```python
from build123d import *

# Parameters (mm, degrees)
BOSS_EXTRUDE1_DEPTH = 37
CUT_EXTRUDE1_REACH  = 186.762
SKETCH2_R           = 11.5
CUT_EXTRUDE2_REACH  = 186.762
SKETCH3_R           = 1.25
SKETCH5_W           = 38
SKETCH5_H           = 23
CUT_EXTRUDE3_DEPTH  = 3
SKETCH6_W           = 3
SKETCH6_H           = 23
BOSS_EXTRUDE2_DEPTH = 7.5
CUT_EXTRUDE4_REACH  = 184.696
SKETCH7_R           = 1.25
SKETCH8_R           = 2.05
CUT_EXTRUDE5_DEPTH  = 2
CUT_EXTRUDE6_REACH  = 181.313
SKETCH9_R           = 2.25
SKETCH10_R          = 3.6
CUT_EXTRUDE7_DEPTH  = 4
CHAMFER1_SIZE       = 30
FILLET4_R           = 20


with BuildPart() as part:
    # Sketch1 → Boss-Extrude1 (new body)
    with BuildSketch(Plane(origin=(0, 0, 0), x_dir=(1, 0, 0), z_dir=(0, 1, 0))):
        Polygon((0, 0), (0, 128), (128, 128), (128, 120), (8, 120), (8, 0), align=None)
    extrude(amount=BOSS_EXTRUDE1_DEPTH)

    # Sketch2 → Cut-Extrude1 (cut, up to next)
    with BuildSketch(Plane(origin=(0, 0, -128), x_dir=(-1, 0, 0), z_dir=(0, 0, -1)), mode=Mode.PRIVATE) as cut_extrude1_sk1:
        with Locations((-112, 18.5)):
            Circle(SKETCH2_R)
    cut_extrude1_tool1 = extrude(cut_extrude1_sk1.sketch, amount=-CUT_EXTRUDE1_REACH, mode=Mode.PRIVATE) & part.part
    add(cut_extrude1_tool1.solids().sort_by_distance((112, 18.5, -128))[0], mode=Mode.SUBTRACT)

    # Sketch3 → Cut-Extrude2 (cut, up to next)
    with BuildSketch(Plane(origin=(0, 0, -128), x_dir=(-1, 0, 0), z_dir=(0, 0, -1)), mode=Mode.PRIVATE) as cut_extrude2_sk1:
        with Locations((-75.86, 10.31)):
            Circle(SKETCH3_R)
    cut_extrude2_tool1 = extrude(cut_extrude2_sk1.sketch, amount=-CUT_EXTRUDE2_REACH, mode=Mode.PRIVATE) & part.part
    # Sketch3 → Cut-Extrude2 (cut, up to next)
    with BuildSketch(Plane(origin=(0, 0, -128), x_dir=(-1, 0, 0), z_dir=(0, 0, -1)), mode=Mode.PRIVATE) as cut_extrude2_sk2:
        with Locations((-105.36, 32.19)):
            Circle(SKETCH3_R)
    cut_extrude2_tool2 = extrude(cut_extrude2_sk2.sketch, amount=-CUT_EXTRUDE2_REACH, mode=Mode.PRIVATE) & part.part
    # Sketch3 → Cut-Extrude2 (cut, up to next)
    with BuildSketch(Plane(origin=(0, 0, -128), x_dir=(-1, 0, 0), z_dir=(0, 0, -1)), mode=Mode.PRIVATE) as cut_extrude2_sk3:
        with Locations((-97.36, 32.19)):
            Circle(SKETCH3_R)
    cut_extrude2_tool3 = extrude(cut_extrude2_sk3.sketch, amount=-CUT_EXTRUDE2_REACH, mode=Mode.PRIVATE) & part.part
    # Sketch3 → Cut-Extrude2 (cut, up to next)
    with BuildSketch(Plane(origin=(0, 0, -128), x_dir=(-1, 0, 0), z_dir=(0, 0, -1)), mode=Mode.PRIVATE) as cut_extrude2_sk4:
        with Locations((-89.36, 32.19)):
            Circle(SKETCH3_R)
    cut_extrude2_tool4 = extrude(cut_extrude2_sk4.sketch, amount=-CUT_EXTRUDE2_REACH, mode=Mode.PRIVATE) & part.part
    # Sketch3 → Cut-Extrude2 (cut, up to next)
    with BuildSketch(Plane(origin=(0, 0, -128), x_dir=(-1, 0, 0), z_dir=(0, 0, -1)), mode=Mode.PRIVATE) as cut_extrude2_sk5:
        with Locations((-81.36, 32.19)):
            Circle(SKETCH3_R)
    cut_extrude2_tool5 = extrude(cut_extrude2_sk5.sketch, amount=-CUT_EXTRUDE2_REACH, mode=Mode.PRIVATE) & part.part
    # Sketch3 → Cut-Extrude2 (cut, up to next)
    with BuildSketch(Plane(origin=(0, 0, -128), x_dir=(-1, 0, 0), z_dir=(0, 0, -1)), mode=Mode.PRIVATE) as cut_extrude2_sk6:
        with Locations((-81.36, 4.81)):
            Circle(SKETCH3_R)
    cut_extrude2_tool6 = extrude(cut_extrude2_sk6.sketch, amount=-CUT_EXTRUDE2_REACH, mode=Mode.PRIVATE) & part.part
    # Sketch3 → Cut-Extrude2 (cut, up to next)
    with BuildSketch(Plane(origin=(0, 0, -128), x_dir=(-1, 0, 0), z_dir=(0, 0, -1)), mode=Mode.PRIVATE) as cut_extrude2_sk7:
        with Locations((-89.36, 4.81)):
            Circle(SKETCH3_R)
    cut_extrude2_tool7 = extrude(cut_extrude2_sk7.sketch, amount=-CUT_EXTRUDE2_REACH, mode=Mode.PRIVATE) & part.part
    # Sketch3 → Cut-Extrude2 (cut, up to next)
    with BuildSketch(Plane(origin=(0, 0, -128), x_dir=(-1, 0, 0), z_dir=(0, 0, -1)), mode=Mode.PRIVATE) as cut_extrude2_sk8:
        with Locations((-97.36, 4.81)):
            Circle(SKETCH3_R)
    cut_extrude2_tool8 = extrude(cut_extrude2_sk8.sketch, amount=-CUT_EXTRUDE2_REACH, mode=Mode.PRIVATE) & part.part
    # Sketch3 → Cut-Extrude2 (cut, up to next)
    with BuildSketch(Plane(origin=(0, 0, -128), x_dir=(-1, 0, 0), z_dir=(0, 0, -1)), mode=Mode.PRIVATE) as cut_extrude2_sk9:
        with Locations((-105.36, 4.81)):
            Circle(SKETCH3_R)
    cut_extrude2_tool9 = extrude(cut_extrude2_sk9.sketch, amount=-CUT_EXTRUDE2_REACH, mode=Mode.PRIVATE) & part.part
    # Sketch3 → Cut-Extrude2 (cut, up to next)
    with BuildSketch(Plane(origin=(0, 0, -128), x_dir=(-1, 0, 0), z_dir=(0, 0, -1)), mode=Mode.PRIVATE) as cut_extrude2_sk10:
        with Locations((-75.86, 26.69)):
            Circle(SKETCH3_R)
    cut_extrude2_tool10 = extrude(cut_extrude2_sk10.sketch, amount=-CUT_EXTRUDE2_REACH, mode=Mode.PRIVATE) & part.part
    add(cut_extrude2_tool1.solids().sort_by_distance((75.86, 10.31, -128))[0], mode=Mode.SUBTRACT)
    add(cut_extrude2_tool2.solids().sort_by_distance((105.36, 32.19, -128))[0], mode=Mode.SUBTRACT)
    add(cut_extrude2_tool3.solids().sort_by_distance((97.36, 32.19, -128))[0], mode=Mode.SUBTRACT)
    add(cut_extrude2_tool4.solids().sort_by_distance((89.36, 32.19, -128))[0], mode=Mode.SUBTRACT)
    add(cut_extrude2_tool5.solids().sort_by_distance((81.36, 32.19, -128))[0], mode=Mode.SUBTRACT)
    add(cut_extrude2_tool6.solids().sort_by_distance((81.36, 4.81, -128))[0], mode=Mode.SUBTRACT)
    add(cut_extrude2_tool7.solids().sort_by_distance((89.36, 4.81, -128))[0], mode=Mode.SUBTRACT)
    add(cut_extrude2_tool8.solids().sort_by_distance((97.36, 4.81, -128))[0], mode=Mode.SUBTRACT)
    add(cut_extrude2_tool9.solids().sort_by_distance((105.36, 4.81, -128))[0], mode=Mode.SUBTRACT)
    add(cut_extrude2_tool10.solids().sort_by_distance((75.86, 26.69, -128))[0], mode=Mode.SUBTRACT)

    # Sketch5 → Cut-Extrude3 (cut)
    with BuildSketch(Plane(origin=(0, 0, -128), x_dir=(-1, 0, 0), z_dir=(0, 0, -1))):
        with Locations((-90, 18.5)):
            Rectangle(SKETCH5_W, SKETCH5_H)
    extrude(amount=-CUT_EXTRUDE3_DEPTH, mode=Mode.SUBTRACT)

    # Sketch6 → Boss-Extrude2 (add)
    with BuildSketch(Plane(origin=(71, 0, 0), x_dir=(0, 0, -1), z_dir=(1, 0, 0))):
        with Locations((126.5, 18.5)):
            Rectangle(SKETCH6_W, SKETCH6_H)
    extrude(amount=BOSS_EXTRUDE2_DEPTH)

    # Sketch7 → Cut-Extrude4 (cut, up to next)
    with BuildSketch(Plane.XY.offset(-125), mode=Mode.PRIVATE) as cut_extrude4_sk1:
        with Locations(Location((75.86, 10.31, 0), (0, 0, 180))):
            Circle(SKETCH7_R)
    cut_extrude4_tool1 = extrude(cut_extrude4_sk1.sketch, amount=-CUT_EXTRUDE4_REACH, mode=Mode.PRIVATE) & part.part
    # Sketch7 → Cut-Extrude4 (cut, up to next)
    with BuildSketch(Plane.XY.offset(-125), mode=Mode.PRIVATE) as cut_extrude4_sk2:
        with Locations(Location((75.86, 26.69, 0), (0, 0, 180))):
            Circle(SKETCH7_R)
    cut_extrude4_tool2 = extrude(cut_extrude4_sk2.sketch, amount=-CUT_EXTRUDE4_REACH, mode=Mode.PRIVATE) & part.part
    add(cut_extrude4_tool1.solids().sort_by_distance((75.86, 10.31, -125))[0], mode=Mode.SUBTRACT)
    add(cut_extrude4_tool2.solids().sort_by_distance((75.86, 26.69, -125))[0], mode=Mode.SUBTRACT)

    # Sketch8 → Cut-Extrude5 (cut)
    with BuildSketch(Plane.XY.offset(-120)):
        with Locations((75.86, 10.31)):
            Circle(SKETCH8_R)
        with Locations((75.86, 26.69)):
            Circle(SKETCH8_R)
        with Locations((81.36, 32.19)):
            Circle(SKETCH8_R)
        with Locations((89.36, 32.19)):
            Circle(SKETCH8_R)
        with Locations((97.36, 32.19)):
            Circle(SKETCH8_R)
        with Locations((105.36, 32.19)):
            Circle(SKETCH8_R)
        with Locations((105.36, 4.81)):
            Circle(SKETCH8_R)
        with Locations((97.36, 4.81)):
            Circle(SKETCH8_R)
        with Locations((89.36, 4.81)):
            Circle(SKETCH8_R)
        with Locations((81.36, 4.81)):
            Circle(SKETCH8_R)
    extrude(amount=-CUT_EXTRUDE5_DEPTH, mode=Mode.SUBTRACT)

    # Sketch9 → Cut-Extrude6 (cut, up to next)
    with BuildSketch(Plane(origin=(8, 0, 0), x_dir=(0, 0, -1), z_dir=(1, 0, 0)), mode=Mode.PRIVATE) as cut_extrude6_sk1:
        with Locations((29, 31)):
            Circle(SKETCH9_R)
    cut_extrude6_tool1 = extrude(cut_extrude6_sk1.sketch, amount=-CUT_EXTRUDE6_REACH, mode=Mode.PRIVATE) & part.part
    # Sketch9 → Cut-Extrude6 (cut, up to next)
    with BuildSketch(Plane(origin=(8, 0, 0), x_dir=(0, 0, -1), z_dir=(1, 0, 0)), mode=Mode.PRIVATE) as cut_extrude6_sk2:
        with Locations((19, 31)):
            Circle(SKETCH9_R)
    cut_extrude6_tool2 = extrude(cut_extrude6_sk2.sketch, amount=-CUT_EXTRUDE6_REACH, mode=Mode.PRIVATE) & part.part
    # Sketch9 → Cut-Extrude6 (cut, up to next)
    with BuildSketch(Plane(origin=(8, 0, 0), x_dir=(0, 0, -1), z_dir=(1, 0, 0)), mode=Mode.PRIVATE) as cut_extrude6_sk3:
        with Locations((9, 31)):
            Circle(SKETCH9_R)
    cut_extrude6_tool3 = extrude(cut_extrude6_sk3.sketch, amount=-CUT_EXTRUDE6_REACH, mode=Mode.PRIVATE) & part.part
    # Sketch9 → Cut-Extrude6 (cut, up to next)
    with BuildSketch(Plane(origin=(8, 0, 0), x_dir=(0, 0, -1), z_dir=(1, 0, 0)), mode=Mode.PRIVATE) as cut_extrude6_sk4:
        with Locations((19, 6)):
            Circle(SKETCH9_R)
    cut_extrude6_tool4 = extrude(cut_extrude6_sk4.sketch, amount=-CUT_EXTRUDE6_REACH, mode=Mode.PRIVATE) & part.part
    # Sketch9 → Cut-Extrude6 (cut, up to next)
    with BuildSketch(Plane(origin=(8, 0, 0), x_dir=(0, 0, -1), z_dir=(1, 0, 0)), mode=Mode.PRIVATE) as cut_extrude6_sk5:
        with Locations((29, 6)):
            Circle(SKETCH9_R)
    cut_extrude6_tool5 = extrude(cut_extrude6_sk5.sketch, amount=-CUT_EXTRUDE6_REACH, mode=Mode.PRIVATE) & part.part
    # Sketch9 → Cut-Extrude6 (cut, up to next)
    with BuildSketch(Plane(origin=(8, 0, 0), x_dir=(0, 0, -1), z_dir=(1, 0, 0)), mode=Mode.PRIVATE) as cut_extrude6_sk6:
        with Locations((9, 6)):
            Circle(SKETCH9_R)
    cut_extrude6_tool6 = extrude(cut_extrude6_sk6.sketch, amount=-CUT_EXTRUDE6_REACH, mode=Mode.PRIVATE) & part.part
    add(cut_extrude6_tool1.solids().sort_by_distance((8, 31, -29))[0], mode=Mode.SUBTRACT)
    add(cut_extrude6_tool2.solids().sort_by_distance((8, 31, -19))[0], mode=Mode.SUBTRACT)
    add(cut_extrude6_tool3.solids().sort_by_distance((8, 31, -9))[0], mode=Mode.SUBTRACT)
    add(cut_extrude6_tool4.solids().sort_by_distance((8, 6, -19))[0], mode=Mode.SUBTRACT)
    add(cut_extrude6_tool5.solids().sort_by_distance((8, 6, -29))[0], mode=Mode.SUBTRACT)
    add(cut_extrude6_tool6.solids().sort_by_distance((8, 6, -9))[0], mode=Mode.SUBTRACT)

    # Sketch10 → Cut-Extrude7 (cut)
    with BuildSketch(Plane(origin=(8, 0, 0), x_dir=(0, 0, -1), z_dir=(1, 0, 0))):
        with Locations((9, 31)):
            Circle(SKETCH10_R)
        with Locations((19, 31)):
            Circle(SKETCH10_R)
        with Locations((29, 31)):
            Circle(SKETCH10_R)
        with Locations((29, 6)):
            Circle(SKETCH10_R)
        with Locations((19, 6)):
            Circle(SKETCH10_R)
        with Locations((9, 6)):
            Circle(SKETCH10_R)
    extrude(amount=-CUT_EXTRUDE7_DEPTH, mode=Mode.SUBTRACT)

    # Chamfer1
    chamfer1_edges = [part.edges().sort_by_distance(p)[0] for p in [
        (8, 18.5, -120),
    ]]
    chamfer(chamfer1_edges, length=CHAMFER1_SIZE)

    # Fillet4
    fillet4_edges = [part.edges().sort_by_distance(p)[0] for p in [
        (38, 18.5, -120),
        (8, 18.5, -90),
    ]]
    fillet(fillet4_edges, radius=FILLET4_R)


solid = part.part
```
The model under review builds one solid part; all positions refer to its coordinate system, in mm. A direction names the side the tool comes from. Round coordinates to 2 decimals unless told otherwise and drop trailing zeros. Order: outer loops, then holes, each group sorted by start corner. A loop starts at its lowest first (then second) coordinate and runs counter-clockwise, first axis right, second up. Notation, with made-up numbers: (-31.5, 72.5) - (9.5, 72.5) arc R27 cw to (9.5, 94.5) - close; hole circle Ø7 at (39.25, 51.25). An arc over 180 degrees is marked (long way). Answer in a Markdown table with one row per item.
(1) Machinability: for faces 4 (the face through (80, 4, -122)), 5 (the face through (91, 19, -125)), 6 (the face through (4, 8, -11)), which of the approach directions +Z, -Z, +X, -X, +Y, -Y give a long, thin tool a straight path to every point of the face, cutting with its end or side? Answer none if there is none.
Result set:
| item | result |
|---|---|
| face 4 | +Z |
| face 5 | -Z |
| face 6 | +X |
(2) Mouldability with a two-part tool opening along X and no side actions: class faces 1 (the face through (9.565, 18.759, -89.471)), 2 (the face through (88, 31, -122)), 3 (the face through (6.03, 34.57, -8.53)) as released by +X, released by -X, zero draft, split by the parting line, or undercut.
Result set:
| item | result |
|---|---|
| face 1 | released by +X |
| face 2 | undercut |
| face 3 | zero draft |
(3) Clearance check with flat-ended pins moving along their axes: P1, Ø2, axis at y = 20.5, z = -80.5, coming from the +X side; P2, Ø3, axis at x = 105.36, y = 4.81, coming from the -Z side; P3, Ø6.5, axis at y = 6, z = -9, coming from the +X side; P4, Ø8, axis at x = 51, y = 17, coming from the +Z side. State where each tip first meets the part, or that it passes through.
Result set:
| item | result |
|---|---|
| P1 | stops at x = 8 |
| P2 | stops at z = -128 |
| P3 | stops at x = 4 |
| P4 | stops at z = -120 |
(4) Take a section at A-A on z = -19. Write out the cut boundary in (x, y), plus the area to 3 significant figures.
Result set:
| item | result |
|---|---|
| outline | (0, 0) - (8, 0) - (8, 2.4) - (4, 2.4) - (4, 3.75) - (0, 3.75) - close; (0, 8.25) - (4, 8.25) - (4, 9.6) - (8, 9.6) - (8, 27.4) - (4, 27.4) - (4, 28.75) - (0, 28.75) - close; (0, 33.25) - (4, 33.25) - (4, 34.6) - (8, 34.6) - (8, 37) - (0, 37) - close |
| area | 202 mm2 |
(5) For line 1 (Y direction, x = 75.86, z = -120.8); line 2 (Y direction, x = 5.9, z = -19); line 3 (Z direction, x = 68, y = 33.5), list the stretches that pass through material, from the lowest coordinate up. Write a range as from..to.
Result set:
| item | result |
|---|---|
| line 1 | y = 0..8.26, 12.36..24.64, 28.74..37 |
| line 2 | y = 0..2.4, 9.6..27.4, 34.6..37 |
| line 3 | z = -128..-120 |
(6) Take a section at D-D on z = -77. Write out the cut boundary in (x, y).
Result set:
| item | result |
|---|---|
| outline | (0, 0) - (8, 0) - (8, 37) - (0, 37) - close |
(7) Take a section at B-B on y = 18.5. Write out the cut boundary in (x, z), plus the area to 3 significant figures.
Result set:
| item | result |
|---|---|
| outline | (0, -128) - (78.5, -128) - (78.5, -125) - (100.5, -125) - (100.5, -120) - (46.28, -120) arc R20 cw to (32.14, -114.14) - (13.86, -95.86) arc R20 cw to (8, -81.72) - (8, 0) - (0, 0) - close; (123.5, -128) - (128, -128) - (128, -120) - (123.5, -120) - close |
| area | 2,200 mm2 |
(8) Take a section at C-C on x = 30.5. Write out the cut boundary in (y, z).
Result set:
| item | result |
|---|---|
| outline | (0, -128) - (37, -128) - (37, -112.5) - (0, -112.5) - close |
